Autodesk Inventor part; units mm, degrees
ref_plane "YZ Plane" through (0, 0, 0) normal (1, 0, 0) x (0, 1, 0)
ref_plane "XZ Plane" through (0, 0, 0) normal (0, 1, 0) x (-1, 0, 0)
ref_plane "XY Plane" through (0, 0, 0) normal (0, 0, 1) x (1, 0, 0)
sketch "Sketch1" plane through (0, 0, 0) normal (0, 0, 1) x (1, 0, 0)
  circle A0 centre (0, 0) radius 19.25
  line L0 (-85, 40) -> (85, 40)
  line L1 (85, 40) -> (85, -30)
  line L2 (85, -30) -> (-85, -30)
  line L3 (-85, -30) -> (-85, 40)
  circle A1 centre (57.5, 0) radius 11.905
  circle A2 centre (-57.5, 0) radius 11.905
  dimension "d0" = 38.5
  dimension "d1" = 23.81
  dimension "d2" = 23.81
  dimension "d3" = 57.5
  dimension "d4" = 57.5
  dimension "d5" = 170
  dimension "d6" = 85
  dimension "d7" = 70
  dimension "d8" = 40
extrude "Extrusion1" add sketch "Sketch1" along normal blind 25.4
sketch "Sketch2" plane through (-85, 40, 0) normal (0, 1, 0) x (1, 0, 0)
  circle A0 centre (85, -12.7) radius 4.215
  line L0 (170, 0) -> (170, -25.4)
  point P0 (85, 0)
  dimension "d11" = 8.43
  dimension "d12" = 12.7
  dimension "d13" = 85
extrude "Extrusion2" cut sketch "Sketch2" against normal blind 25.4
properties part number "1234_Spool Plate_V1" material "Aluminum"
Build history of the part. All positions in model axes, mm. A direction names the side the tool comes from. Coordinates: 2 decimals unless noted, no trailing zeros. Order: outer loops, then holes, each group sorted by start corner. A loop starts at its lowest first (then second) coordinate and runs counter-clockwise, first axis right, second up. Notation, with made-up numbers: (-18, 5.25) -> (23, 5.25) arc R13 cw to (23, 25.25) -> close; hole circle Ø8 at (0, 83). An arc over 180 degrees is marked (long way). Answer in a Markdown table with one row per item. Add a question column.
Q1. Band-saw the part on B-B, the plane y = 0. List the corners of the cut face in (x, z) (3 decimals).
Q2. Band-saw the part on A-A, the plane x = 0. List the corners of the cut face in (y, z) (3 decimals), then the cut area to 3 significant figures.
Q3. Wall check: line 1 along X through (y, z) = (-9.5, 7.25); line 2 along Z through (x, y) = (0, 27.25) (3 decimals); line 3 along X through (y, z) = (11, 4). Give the ranges that are in metal, low to high. Write a range as [from, to].
Q4. Which spindle directions (+Z, -Z, +X, -X, +Y, -Y) get a long thin tool onto all of the face, cutting with end or side? Do faces 4 (the face through (2.27, 29.54, 9.15)), 5 (the face through (-1, 40, 18)). Say none if no direction does.
Q5. Mould opens along Y. For faces 1 (the face through (1, -30, 13)), 2 (the face through (-85, 5, 13)), 3 (the face through (10.35, -16.23, 12.52)) say: +Y half, -Y half, draft (parallel to the pull), parting line (faces both ways), or undercut.
Q6. Drop a flat-ended pin along its axis: pin 1 (14.5 mm diameter, centred on x = 57.5, y = 0, fed in from +Z). Give the stop position or say it passes through.
Q7. Band-saw the part on D-D, the plane z = 12.7. List the corners of the cut face in (x, y) (3 decimals), then the cut area to 3 significant figures.
Q8. Band-saw the part on C-C, the plane z = 19.5. List the corners of the cut face in (x, y) (3 decimals), then the cut area to 3 significant figures.
Answers follow:
| question | item | result |
|---|---|---|
| 1 | outline | (-85, 0) -> (-69.405, 0) -> (-69.405, 25.4) -> (-85, 25.4) -> close; (-45.595, 0) -> (-19.25, 0) -> (-19.25, 25.4) -> (-45.595, 25.4) -> close; (19.25, 0) -> (45.595, 0) -> (45.595, 25.4) -> (19.25, 25.4) -> close; (69.405, 0) -> (85, 0) -> (85, 25.4) -> (69.405, 25.4) -> close |
| 2 | outline | (-30, 0) -> (-19.25, 0) -> (-19.25, 25.4) -> (-30, 25.4) -> close; (19.25, 0) -> (40, 0) -> (40, 8.485) -> (19.25, 8.485) -> close; (19.25, 16.915) -> (40, 16.915) -> (40, 25.4) -> (19.25, 25.4) -> close |
| 2 | area | 625 mm^2 |
| 3 | line 1 | [-85, -64.67], [-50.33, -16.74], [16.74, 50.33], [64.67, 85] |
| 3 | line 2 | [0, 8.485], [16.915, 25.4] |
| 3 | line 3 | [-85, -62.05], [-52.95, -15.8], [15.8, 52.95], [62.05, 85] |
| 4 | face 4 | +Y |
| 4 | face 5 | +Z, -Z, +X, -X, +Y |
| 5 | face 1 | -Y half |
| 5 | face 2 | draft |
| 5 | face 3 | undercut |
| 6 | pin 1 | through |
| 7 | outline | (-85, -30) -> (85, -30) -> (85, 40) -> (4.215, 40) -> (4.215, 18.783) arc R19.25 cw (long way) to (-4.215, 18.783) -> (-4.215, 40) -> (-85, 40) -> close; hole circle Ø23.81 at (-57.5, 0); hole circle Ø23.81 at (57.5, 0) |
| 7 | area | 9,670 mm^2 |
| 8 | outline | (-85, -30) -> (85, -30) -> (85, 40) -> (-85, 40) -> close; hole circle Ø23.81 at (-57.5, 0); hole circle Ø38.5 at (0, 0); hole circle Ø23.81 at (57.5, 0) |
| 8 | area | 9,850 mm^2 |
